```python
from build123d import *

# Parameters (mm, degrees)
SKETCH9_R           = 25
BOSS_EXTRUDE1_DEPTH = 125
SKETCH10_R          = 12.5
BOSS_EXTRUDE4_DEPTH = 150
SKETCH20_R          = 2.5
CUT_EXTRUDE5_DEPTH  = 20
SKETCH19_R          = 2.5
CUT_EXTRUDE6_DEPTH  = 20


with BuildPart() as part:
    # Sketch9 → Boss-Extrude1 (new body, symmetric)
    with BuildSketch(Plane.XY):
        Circle(SKETCH9_R)
    extrude(amount=BOSS_EXTRUDE1_DEPTH, both=True)

    # Sketch10 → Boss-Extrude4 (add, symmetric)
    with BuildSketch(Plane.XY):
        Circle(SKETCH10_R)
    extrude(amount=BOSS_EXTRUDE4_DEPTH, both=True)

    # Sketch20 → Cut-Extrude5 (cut)
    with BuildSketch(Plane(origin=(0, 0, -150), x_dir=(-1, 0, 0), z_dir=(0, 0, -1))):
        with Locations((0, 4.91077603)):
            Circle(SKETCH20_R)
    extrude(amount=-CUT_EXTRUDE5_DEPTH, mode=Mode.SUBTRACT)

    # Sketch19 → Cut-Extrude6 (cut)
    with BuildSketch(Plane.XY.offset(150)):
        with Locations((0, 4.91077603)):
            Circle(SKETCH19_R)
    extrude(amount=-CUT_EXTRUDE6_DEPTH, mode=Mode.SUBTRACT)


solid = part.part
```
Model file for the job. Use its own axes, mm. A direction names the side the tool comes from. Round coordinates to 2 decimals unless told otherwise and drop trailing zeros. Order: outer loops, then holes, each group sorted by start corner. A loop starts at its lowest first (then second) coordinate and runs counter-clockwise, first axis right, second up. Notation, with made-up numbers: (8, 62) -> (63, 62) arc R19 cw to (63, 71) -> close; hole circle Ø6 at (-27.75, 69). An arc over 180 degrees is marked (long way). Use one line per item in the form item = value.
Item 1: Cut at A-A, the plane x = 0. Write the cut outline in (y, z).
Returned:
outline = (-25, -125) -> (-12.5, -125) -> (-12.5, -150) -> (2.41, -150) -> (2.41, -130) -> (7.41, -130) -> (7.41, -150) -> (12.5, -150) -> (12.5, -125) -> (25, -125) -> (25, 125) -> (12.5, 125) -> (12.5, 150) -> (7.41, 150) -> (7.41, 130) -> (2.41, 130) -> (2.41, 150) -> (-12.5, 150) -> (-12.5, 125) -> (-25, 125) -> close
Item 2: Tool access for faces 1 (the face through (11.923, 3.755, -137.325)), 2 (the face through (-11.5, 5.9, 125)), 3 (the face through (0, 0, -150)): list every direction of +Z, -Z, +X, -X, +Y, -Y with a clear straight run to the whole face (end or side of a thin tool).
Returned:
face_1 = -Z
face_2 = +Z
face_3 = -Z, +X, -X, +Y, -Y
Item 3: Pull direction Y, two halves, no side cores. Call faces 4 (the face through (11.923, 3.755, 137.675)), 5 (the face through (-0.33, 7.39, 140.14)), 6 (the face through (0, 0, 150)): released by +Y, released by -Y, zero draft, split by the parting line, or undercut.
Returned:
face_4 = split by the parting line
face_5 = undercut
face_6 = zero draft
Item 4: Drill centre lines: line 1 (Y direction, x = 0, z = 140); line 2 (Z direction, x = -10, y = -9); line 3 (Y direction, x = 23, z = -73.5). Where is each one in solid material? Low to high.
Returned:
line_1 = -12.5 to 2.41, 7.41 to 12.5
line_2 = -125 to 125
line_3 = -9.8 to 9.8
Item 5: Cut at B-B, the plane y = -7. Write the cut outline in (x, z).
Returned:
outline = (-24, -125) -> (-10.36, -125) -> (-10.36, -150) -> (10.36, -150) -> (10.36, -125) -> (24, -125) -> (24, 125) -> (10.36, 125) -> (10.36, 150) -> (-10.36, 150) -> (-10.36, 125) -> (-24, 125) -> close
Item 6: Cut at C-C, the plane z = 91. Write the cut outline in (x, y), and give its area (3 significant figures).
Returned:
outline = circle Ø50 at (0, 0)
area = 1,960 mm^2
Item 7: Cut at D-D, the plane x = -20. Write the cut outline in (y, z).
Returned:
outline = (-15, -125) -> (15, -125) -> (15, 125) -> (-15, 125) -> close
Item 8: Flat gauge pins, fed straight in: pin 1 Ø1 at (x, z) = (-2.5, 96.5) entering from -Y; pin 2 Ø4 at (x, y) = (0, 4.91) entering from +Z; pin 3 Ø1 at (y, z) = (16.5, 29.5) entering from -X. Where does each tip first touch, or does it go through?
Returned:
pin_1 = -24.92
pin_2 = 130
pin_3 = -19.21
